Build history of the part. All positions in model axes, mm. A direction names the side the tool comes from. Give positions to 0.01 mm unless a question says otherwise; leave off trailing zeros. Write each loop counter-clockwise with the first axis right and the second up, starting at its lowest first coordinate (ties: lowest second). Pieces come first, ordered by that corner, then holes. Notation, with made-up numbers: (78.5, 20) -> (130.5, 20) arc R29 ccw to (130.5, 53) -> close; hole circle Ø1 at (-38, -31). An arc over 180 degrees is marked (long way). Write item = value, one per line. Start each with the question number.
Q1. Drop flat-ended pins along their axis: P1, Ø3, axis at x = -34.5, z = 28.5, coming from the -Y side; P2, Ø1.5, axis at x = 12.5, z = 14, coming from the +Y side; P3, Ø4, axis at x = -7, z = 8.5, coming from the +Y side. Give the stop position or say it passes through.
Q2. Mould opens along X. For faces 1 (the face through (61.617, -13, 25)), 2 (the face through (5.688, 22.591, 40.597)), 3 (the face through (5, 0, 0)) say: pulls with the +X half, pulls with the -X half, needs draft (parallel to the pull), parting line crosses it, or undercut.
Q3. Saw through at B-B, the plane y = -4. List the corners of the cut face in (x, z).
Q4. Saw through at C-C, the plane z = 36. List the corners of the cut face in (x, y), then the cut area to 3 significant figures.
Q5. Tool access for faces 4 (the face through (5.947, -21.939, 40.597)), 5 (the face through (-50.171, -13, 25)), 6 (the face through (5.35, -35.11, 33.71)): list every direction of +Z, -Z, +X, -X, +Y, -Y with a clear straight run to the whole face (end or side of a thin tool).
Q6. Saw through at D-D, the plane y = -22. List the corners of the cut face in (x, z), then the cut area to 3 significant figures.
Q7. Saw through at A-A, the plane z = 45.5. List the corners of the cut face in (x, y).
Q8. Wall check: line 1 (X direction, y = -25, z = 12.5); line 2 (X direction, y = -0.5, z = 18); line 3 (Y direction, x = -9, z = 38.5). Give the ranges that are in metal, low to high.
from build123d import *
from build123d import SkipClean  # not in build123d's __all__

# Parameters (mm, degrees)
F1_DEPTH = 50.8
F3_DEPTH = 33.782
F4_DEPTH = 19.304
F7_DEPTH = 62.738
F8_DEPTH = 50.8


with BuildPart() as f1:
    # F0 (on Top) → F1 (new body)
    with BuildSketch(Plane.XY):
        Polygon((-50.1712188125, 0), (-50.1712188125, -25.5924221128), (61.6167448461, -25.5924221128), (61.6167448461, 0.6504831836), align=None)
    extrude(amount=F1_DEPTH)

    # F2 (on face) → F3 (cut)
    with BuildSketch(Plane.XZ.offset(25.5924221128)):
        with BuildLine():
            Line((15.9283644421, 50.8), (-4.4828384085, 50.8))
            ThreePointArc((-4.4828384085, 50.8), (5.7227630168, 40.5943985747), (15.9283644421, 50.8))
        make_face()
    extrude(amount=-F3_DEPTH, mode=Mode.SUBTRACT)

    # F2 (on face) → F4 (join)
    with BuildSketch(Plane.XZ.offset(25.5924221128)):
        with BuildLine():
            Line((-4.4828384085, 50.8), (-11.371643244, 50.8))
            ThreePointArc((-11.371643244, 50.8), (5.7227630168, 33.7055937392), (22.8171692776, 50.8))
            Line((22.8171692776, 50.8), (15.9283644421, 50.8))
            ThreePointArc((15.9283644421, 50.8), (5.7227630168, 40.5943985747), (-4.4828384085, 50.8))
        make_face()
    extrude(amount=F4_DEPTH)

    # F5 (on face) → F7 (cut)
    with BuildSketch(Plane.XY.offset(50.8)):
        with BuildLine():
            Line((-20.977136112, 0.1698775005), (-33.6769211089, 0.0959786987))
            ThreePointArc((-33.6769211089, 0.0959786987), (-27.2900792096, -6.2169643988), (-20.977136112, 0.1698775005))
        make_face()
    extrude(amount=-F7_DEPTH, mode=Mode.SUBTRACT)

    # F6 (on face) → F8 (cut)
    with BuildSketch(Plane.XY.offset(50.8)):
        with BuildLine():
            Line((45.1224471426, 0.5545044849), (32.4226621457, 0.480605683))
            ThreePointArc((32.4226621457, 0.480605683), (38.809504045, -5.8323374145), (45.1224471426, 0.5545044849))
        make_face()
    extrude(amount=-F8_DEPTH, mode=Mode.SUBTRACT)

    # F9: F1 across face


with BuildPart() as f1_1:
    add(f1.part, clean=False)
    with SkipClean():  # cleaning this boolean's faces spoils the solid; the shape is the same uncleaned
        add(f1.part.mirror(Plane(origin=(5.7227630168, 0.3252415918, 24.0477864572), x_dir=(-0.9999830706, -0.0058188033, 0), z_dir=(-0.0058188033, 0.9999830706, 0))), clean=False)


solid = f1_1.part
Report:
q1.P1 = -25.59
q1.P2 = 26.33
q1.P3 = 26.12
q2.face_1 = pulls with the +X half
q2.face_2 = undercut
q2.face_3 = needs draft
q3.outline = (-50.17, 0) -> (-32.15, 0) -> (-32.15, 50.8) -> (-50.17, 50.8) -> close; (-22.51, 0) -> (34.31, 0) -> (34.31, 50.8) -> (15.93, 50.8) arc R10.21 cw to (-4.48, 50.8) -> (-22.51, 50.8) -> close; (43.24, 0) -> (61.62, 0) -> (61.62, 50.8) -> (43.24, 50.8) -> close
q4.outline = (-50.47, 25.59) -> (-50.17, 0) -> (-50.17, -25.59) -> (-2.83, -25.59) -> (-2.83, -44.9) -> (14.28, -44.9) -> (14.28, -25.59) -> (61.62, -25.59) -> (61.62, 0.65) -> (61.31, 26.89) -> (13.98, 26.34) -> (13.75, 45.64) -> (-3.36, 45.44) -> (-3.13, 26.14) -> close; hole circle Ø12.7 at (-27.33, 0.13); hole circle Ø12.7 at (38.77, 0.52)
q4.area = 6,200 mm2
q5.face_4 = +Z, -Y
q5.face_5 = +Z, -Z, -X, -Y
q5.face_6 = -Z, -Y
q6.outline = (-50.17, 0) -> (61.62, 0) -> (61.62, 50.8) -> (15.93, 50.8) arc R10.21 cw to (-4.48, 50.8) -> (-50.17, 50.8) -> close
q6.area = 5,520 mm2
q7.outline = (-50.47, 25.59) -> (-50.17, 0) -> (-50.17, -25.59) -> (-10.53, -25.59) -> (-10.53, -44.9) -> (-3, -44.9) -> (-3, 0.27) -> (-3.52, 45.44) -> (-11.05, 45.35) -> (-10.83, 26.05) -> close; (13.92, 45.65) -> (14.44, 0.38) -> (14.44, -44.9) -> (21.97, -44.9) -> (21.97, -25.59) -> (61.62, -25.59) -> (61.62, 0.65) -> (61.31, 26.89) -> (21.67, 26.43) -> (21.45, 45.73) -> close; hole circle Ø12.7 at (-27.33, 0.13); hole circle Ø12.7 at (38.77, 0.52)
q8.line_1 = -50.17 to 61.62
q8.line_2 = -50.17 to -33.65, -21.01 to 32.5, 45.04 to 61.62
q8.line_3 = -25.59 to 26.07
